Study the drawing (mm; zero at the part's minimum x, y, z) and answer. A direction names the side the tool comes from. Coordinates: 2 decimals unless noted, no trailing zeros. Write each loop counter-clockwise with the first axis right and the second up, starting at its lowest first coordinate (ties: lowest second). Pieces come first, ordered by that corner, then holes. Notation, with made-up numbers: (14, -38) -> (49, -38) arc R31 ccw to (49, -12) -> close; hole circle Ø8 at (-11, 35). An arc over 180 degrees is marked (long way). Answer in a Markdown table with one row per item. Add a question column.
Item 1: Given pin 1 Ø6 at (x, z) = (16, 11.5) entering from +Y; pin 2 Ø4 at (y, z) = (70, 26) entering from -X; pin 3 Ø12 at (x, y) = (15, 22.5) entering from +Z, each flat-ended and moving along its own axis, determine where each tip first touches the part or whether it passes through.
Item 2: Which of the six approach directions +Z, -Z, +X, -X, +Y, -Y give full straight-line access (tool end or side, diameter ignored) to the marked faces 1 and 2?
Item 3: Straight lines are drawn through the part: line 1 (Y direction, x = 15, z = 35); line 2 (Y direction, x = 8, z = 12); line 3 (Z direction, x = 7, y = 55). For each, find the intervals that lie inside material, in ascending order. Write a range as from..to.
Item 4: Section B-B on z = 15 is taken. Write down the section's boundary in (x, y).
Item 5: Section C-C on y = 65 is taken. Write down the section's boundary in (x, z), then the cut area to 3 significant figures.
Item 6: Section D-D on x = 20 is taken. Write down the section's boundary in (y, z).
Item 7: Section A-A on x = 13 is taken. Write down the section's boundary in (y, z).
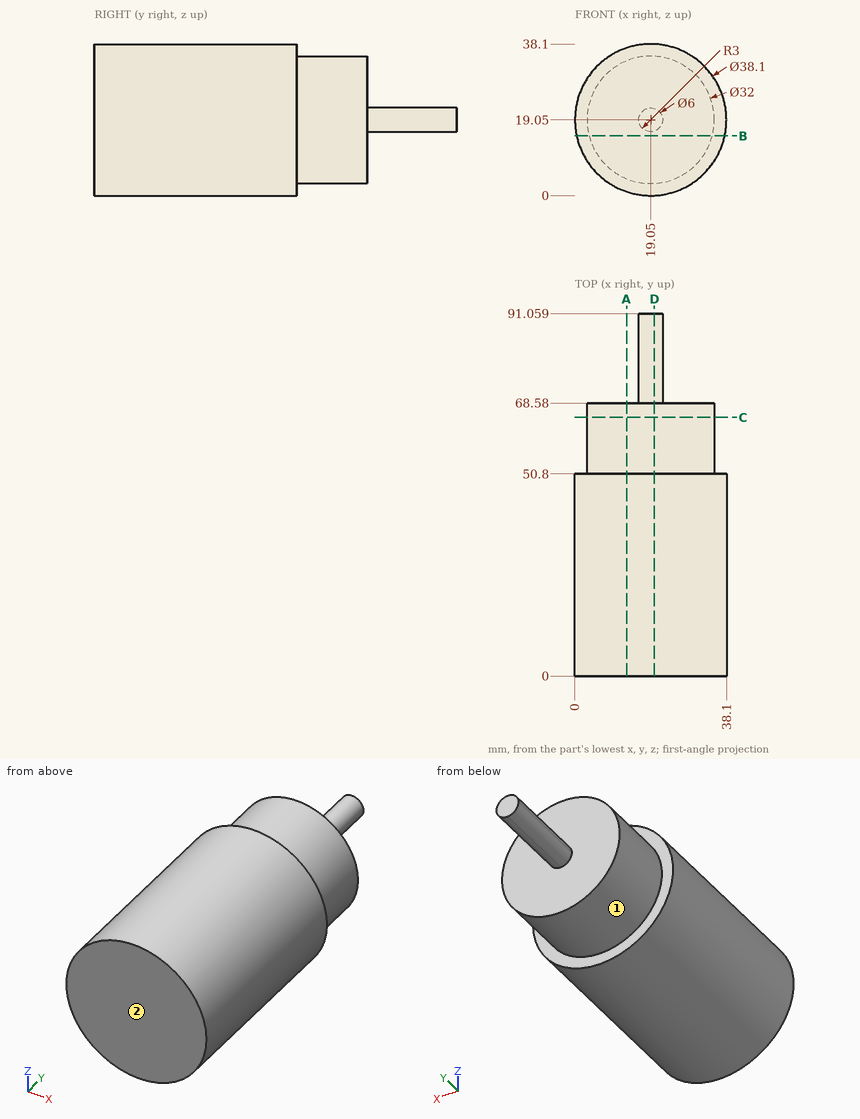
Results below:
| question | item | result |
|---|---|---|
| 1 | pin 1 | stops at y = 68.58 |
| 1 | pin 2 | stops at x = 4.04 |
| 1 | pin 3 | stops at z = 38.1 |
| 2 | face 1 | +Y |
| 2 | face 2 | +Z, -Z, +X, -X, -Y |
| 3 | line 1 | y = 0..50.8 |
| 3 | line 2 | y = 0..68.58 |
| 3 | line 3 | z = 8.52..29.58 |
| 4 | outline | (0.44, 0) -> (37.66, 0) -> (37.66, 50.8) -> (34.53, 50.8) -> (34.53, 68.58) -> (3.57, 68.58) -> (3.57, 50.8) -> (0.44, 50.8) -> close |
| 5 | outline | circle Ø32 at (19.05, 19.05) |
| 5 | area | 804 mm2 |
| 6 | outline | (0, 0.02) -> (50.8, 0.02) -> (50.8, 3.08) -> (68.58, 3.08) -> (68.58, 16.2) -> (91.06, 16.2) -> (91.06, 21.9) -> (68.58, 21.9) -> (68.58, 35.02) -> (50.8, 35.02) -> (50.8, 38.08) -> (0, 38.08) -> close |
| 7 | outline | (0, 0.99) -> (50.8, 0.99) -> (50.8, 4.24) -> (68.58, 4.24) -> (68.58, 33.86) -> (50.8, 33.86) -> (50.8, 37.11) -> (0, 37.11) -> close |
